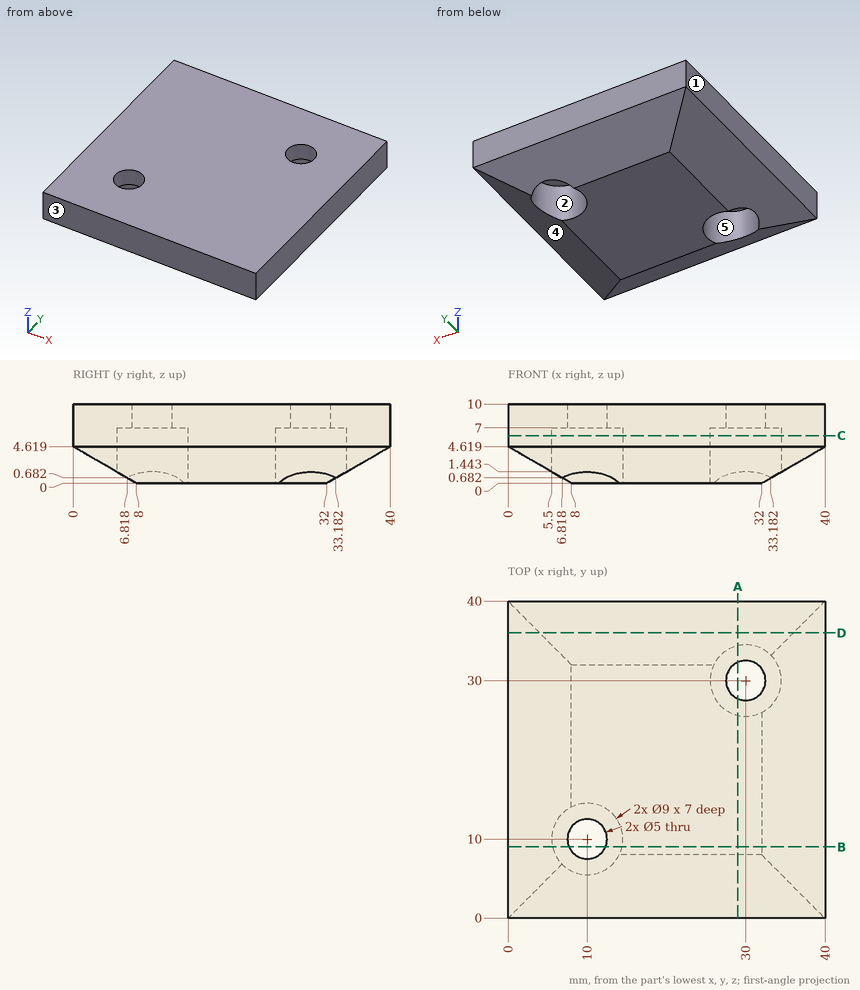
Verification items for this drawing (mm, ordinates from the low corner). A direction names the side the tool comes from. Give positions to 0.01 mm unless a question says otherwise; leave off trailing zeros. Order: outer loops, then holes, each group sorted by start corner. A loop starts at its lowest first (then second) coordinate and runs counter-clockwise, first axis right, second up.
1) Cross-section at C-C (z = 6). Record the boundary of the cut face in (x, y), then the cut area to 3 significant figures.
Results are:
outline: (0, 0) - (40, 0) - (40, 40) - (0, 40) - close; hole circle Ø9 at (10, 10); hole circle Ø9 at (30, 30)
area: 1,470 mm2
2) Draft check along Y on the marked faces 1, 2 and 3. Enter one of: released by +Y, released by -Y, zero draft, split by the parting line, or undercut.
Results are:
face 1: zero draft
face 2: undercut
face 3: released by -Y
3) Cross-section at B-B (y = 9). Record the boundary of the cut face in (x, z).
Results are:
outline: (0, 4.62) - (5.61, 1.38) - (5.61, 7) - (7.71, 7) - (7.71, 10) - (0, 10) - close; (12.29, 7) - (14.39, 7) - (14.39, 0) - (32, 0) - (40, 4.62) - (40, 10) - (12.29, 10) - close
4) Tool access check on the marked faces 4 and 5. Record the directions out of +Z, -Z, +X, -X, +Y, -Y that give a thin tool (end or side, any length) a straight path to the whole face; none if there is none.
Results are:
face 4: -Z, +X, +Y, -Y
face 5: -Z
5) Material ranges on probe 1 along Y at (x, z) = (30, 8.9); probe 2 along Z at (x, y) = (10, 6); probe 3 along Y at (x, z) = (30, 5.75), recorded low to high.
Results are:
probe 1: y = 0 to 27.5, 32.5 to 40
probe 2: z = 7 to 10
probe 3: y = 0 to 25.5, 34.5 to 40
6) Cross-section at D-D (y = 36). Record the boundary of the cut face in (x, z).
Results are:
outline: (0, 4.62) - (4, 2.31) - (36, 2.31) - (40, 4.62) - (40, 10) - (0, 10) - close
7) Cross-section at A-A (x = 29). Record the boundary of the cut face in (y, z).
Results are:
outline: (0, 4.62) - (8, 0) - (25.61, 0) - (25.61, 7) - (27.71, 7) - (27.71, 10) - (0, 10) - close; (32.29, 7) - (34.39, 7) - (34.39, 1.38) - (40, 4.62) - (40, 10) - (32.29, 10) - close
8) Gauge pin test, flat ends, axial feed: pin 1 (1.5 mm diameter, centred on x = 19.5, z = 3.5, fed in from -Y); pin 2 (4 mm diameter, centred on y = 13, z = 2.5, fed in from -X) (1 decimal). Record the tip position at first contact, or that the pin passes through.
Results are:
pin 1: stops at y = 0.64
pin 2: stops at x = 0.2
